CAD build for the part. Positions are in the model's coordinates, mm. Face numbers are marked on the shaded views. Give positions to 0.01 mm unless a question says otherwise; leave off trailing zeros. Loops run counter-clockwise (first coordinate to the right, second up) from the corner with the lowest first, then second, coordinate; pieces in that order, holes last. Notation, with made-up numbers: (19, -40) - (29, -40) arc R22 ccw to (29, -8) - close; hole circle Ø9 at (-25.5, 12.25). An arc over 180 degrees is marked (long way). Return JSON: item names as keys, results as strings.
from build123d import *

# Parameters (mm, degrees)
Y_KSEKLIK_EKSTR_ZYON1_DEPTH = 15
IZIM2_R                     = 1.7
KES_EKSTR_ZYON2_DEPTH       = 15
RADYUS3_R                   = 6.3
IZIM3_R                     = 3
KES_EKSTR_ZYON3_DEPTH       = 15


with BuildPart() as part:
    # Çizim1 → Yükseklik-Ekstrüzyon1 (new body)
    with BuildSketch(Plane.XY):
        with BuildLine():
            Line((-19.5, 0), (-11.225, 0))
            ThreePointArc((-11.225, 0), (0, 11.225), (11.225, 0))
            Line((11.225, 0), (19.5, 0))
            Line((19.5, 0), (19.5, 5))
            Line((19.5, 5), (15.435369286, 5))
            ThreePointArc((15.435369286, 5), (0, 16.225), (-15.435369286, 5))
            Line((-15.435369286, 5), (-19.5, 5))
            Line((-19.5, 5), (-19.5, 0))
        make_face()
    extrude(amount=Y_KSEKLIK_EKSTR_ZYON1_DEPTH)

    # Çizim2 → Kes-Ekstrüzyon2 (cut)
    with BuildSketch(Plane.XZ):
        with Locations((-15, 7.5)):
            Circle(IZIM2_R)
        with Locations((15, 7.5)):
            Circle(IZIM2_R)
    extrude(amount=-KES_EKSTR_ZYON2_DEPTH, mode=Mode.SUBTRACT)

    # Radyus3
    # the kernel refuses this fillet: 6.3 mm, written as the material it adds along each edge
    with BuildSketch(Plane(origin=(-15.435369286, 5, -0.982079778), x_dir=(-1, 0, 0), z_dir=(0, 0, 1))) as radyus3_piece_1_section:
        with BuildLine():
            CenterArc((4.050154186, -6.3), RADYUS3_R, 90, 59.889795344)
            ThreePointArc((-1.399736951, -3.139511654), (-0.61649222, -1.60692875), (0, 0))
            Line((0, 0), (4.050154186, 0))
        make_face()
    radyus3_piece_1 = extrude(amount=15.982079778, mode=Mode.PRIVATE)
    radyus3_piece_1 = split(radyus3_piece_1, bisect_by=Plane(origin=(-18.387347424, 5.060237856, 0), z_dir=(0, 0, 1)), keep=Keep.TOP, mode=Mode.PRIVATE)
    radyus3_piece_1 = radyus3_piece_1 - Plane(origin=(-15, 5.060237856, 7.5), x_dir=(1, 0, 0), z_dir=(0, -1, 0)) * Cylinder(1.7, 49, mode=Mode.PRIVATE)
    add(radyus3_piece_1)
    with BuildSketch(Plane(origin=(15.435369286, 5, -0.982079778), x_dir=(-0.4072067026202576, 0.9133360287107571, 0), z_dir=(0, 0, 1))) as radyus3_piece_2_section:
        with BuildLine():
            CenterArc((4.10476705, -6.264553967), RADYUS3_R, 96.080720065, 59.889795344)
            Line((-1.649249931, -3.69915174), (0, 0))
            ThreePointArc((0, 0), (1.718705687, -0.091287601), (3.437411374, 0))
        make_face()
    radyus3_piece_2 = extrude(amount=15.982079778, mode=Mode.PRIVATE)
    radyus3_piece_2 = split(radyus3_piece_2, bisect_by=Plane(origin=(14.638658108, 7.219740405, 0), z_dir=(0, 0, 1)), keep=Keep.TOP, mode=Mode.PRIVATE)
    radyus3_piece_2 = radyus3_piece_2 - Plane(origin=(15, 7.219740405, 7.5), x_dir=(1, 0, 0), z_dir=(0, -1, 0)) * Cylinder(1.7, 47, mode=Mode.PRIVATE)
    add(radyus3_piece_2)

    # Çizim3 → Kes-Ekstrüzyon3 (cut)
    with BuildSketch(Plane(origin=(0, 5, 0), x_dir=(1, 0, 0), z_dir=(0, 1, 0))):
        with Locations(Location((-15, -7.5, 0), (0, 0, 71.249080341))):
            Circle(IZIM3_R)
        with Locations(Location((15, -7.5, 0), (0, 0, 108.750992195))):
            Circle(IZIM3_R)
    extrude(amount=KES_EKSTR_ZYON3_DEPTH, mode=Mode.SUBTRACT)


solid = part.part
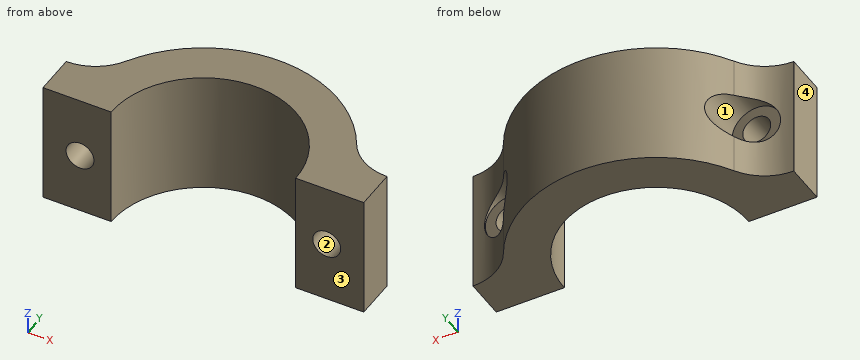
1. Drill centre lines: probe 1 along Z at (x, y) = (-15, 1.7); probe 2 along Z at (x, y) = (15, 6.3); probe 3 along X at (y, z) = (9, 11.5). Where is each one in solid material? Low to high.
Values follow:
{"probe 1": "z = 0 to 5.8, 9.2 to 15", "probe 2": "z = 0 to 4.5, 10.5 to 15", "probe 3": "x = -13.5 to -6.71, 6.71 to 13.5"}
2. Pull direction X, two halves, no side cores. Call the marked faces 1, 2, 3 and 4: +X half, -X half, draft (parallel to the pull), parting line (faces both ways), or undercut.
Values follow:
{"face 1": "undercut", "face 2": "undercut", "face 3": "draft", "face 4": "-X half"}
3. Drop flat-ended pins along their axis: P1, Ø1.5, axis at y = 11.5, z = 10, coming from the -X side; P2, Ø5, axis at x = -3, z = 12.5, coming from the +Y side; P3, Ø1.8, axis at x = -16.5, z = 7.5, coming from the +Y side. Give the stop position or say it passes through.
Values follow:
{"P1": "stops at x = -12.15", "P2": "stops at y = 16.22", "P3": "stops at y = 5"}
4. Cut at B-B, the plane z = 6.75. Write the cut outline in (x, y) (3 decimals).
Values follow:
{"outline": "(-19.5, 0) - (-16.526, 0) - (-16.526, 5) - (-17.905, 5) - (-17.905, 5.202) arc R6.3 cw to (-19.486, 5) - (-19.5, 5) - close; (-13.474, 0) - (-11.225, 0) arc R11.225 cw to (11.225, 0) - (13.474, 0) - (13.474, 5) - (12.095, 5) - (12.095, 10.815) arc R16.225 ccw to (-12.095, 10.815) - (-12.095, 5) - (-13.474, 5) - close; (16.526, 0) - (19.5, 0) - (19.5, 5) - (19.486, 5) arc R6.3 cw to (17.905, 5.202) - (17.905, 5) - (16.526, 5) - close"}
5. Cut at D-D, the plane y = 9.25. Write the cut outline in (x, z).
Values follow:
{"outline": "(-13.33, 0) - (-6.36, 0) - (-6.36, 15) - (-13.33, 15) - (-13.33, 9.99) arc R3 cw to (-13.33, 5.01) - close; (6.36, 0) - (13.33, 0) - (13.33, 5.01) arc R3 cw to (13.33, 9.99) - (13.33, 15) - (6.36, 15) - close"}
6. Cut at A-A, the plane y = 1.5. Write the cut outline in (x, z).
Values follow:
{"outline": "(-19.5, 0) - (-11.12, 0) - (-11.12, 15) - (-19.5, 15) - close; (11.12, 0) - (19.5, 0) - (19.5, 15) - (11.12, 15) - close; hole circle Ø3.4 at (-15, 7.5); hole circle Ø3.4 at (15, 7.5)"}
7. Cut at C-C, the plane x = -15. Write the cut outline in (y, z).
Values follow:
{"outline": "(0, 0) - (6.88, 0) - (6.88, 4.5) - (5, 4.5) - (5, 5.8) - (0, 5.8) - close; (0, 9.2) - (5, 9.2) - (5, 10.5) - (6.88, 10.5) - (6.88, 15) - (0, 15) - close"}
